Build history of the part. All positions in model axes, mm. Round coordinates to 2 decimals unless told otherwise and drop trailing zeros. Loops run counter-clockwise (first coordinate to the right, second up) from the corner with the lowest first, then second, coordinate; pieces in that order, holes last. Notation, with made-up numbers: (31.5, -39.5) - (78.5, -39.5) arc R20 cw to (78.5, -16.5) - close; hole circle Ø1 at (6.5, 76). An arc over 180 degrees is marked (long way). Use one line per item in the form item = value. Start each with the question number.
Q1. Drill centre lines: line 1 (X direction, y = -116, z = 0.6); line 2 (Y direction, x = 55, z = 0.75); line 3 (Y direction, x = 65, z = 1.3). Where is each one in solid material? Low to high.
Q2. Saw through at A-A (x = 65). Give the cut face in (y, z), then the cut area to 3 significant figures.
Q3. Pin check, flat tips, straight feed: pin 1 (9 mm diameter, centred on x = 65, y = -70, fed in from +Z); pin 2 (4.5 mm diameter, centred on x = 55, y = -116, fed in from +Z). Stop position of each tip, or through.
Autodesk Inventor part; units mm, degrees
ref_plane "YZ Plane" through (0, 0, 0) normal (1, 0, 0) x (0, 1, 0)
ref_plane "XZ Plane" through (0, 0, 0) normal (0, 1, 0) x (-1, 0, 0)
ref_plane "XY Plane" through (0, 0, 0) normal (0, 0, 1) x (1, 0, 0)
sketch "スケッチ1" plane through (0, 0, 0) normal (0, 0, 1) x (1, 0, 0)
  line L0 (0, 0) -> (360, 0)
  line L1 (360, 0) -> (360, -180)
  line L2 (360, -180) -> (0, -180)
  line L3 (0, -180) -> (0, 0)
  dimension "d0" = 360
  dimension "d1" = 180
extrude "押し出し1" add sketch "スケッチ1" along normal blind 2
sketch "スケッチ3" plane through (0, 0, 2) normal (0, 0, 1) x (1, 0, 0)
  line L0 (360, 0) -> (0, 0)
  line L1 (0, 0) -> (0, -180)
  point P0 (55, -139)
  point P1 (30, -139)
  point P2 (55, -116)
  point P3 (30, -116)
  dimension "d14" = 139
  dimension "d15" = 55
  dimension "d18" = 25
  dimension "d21" = 23
hole "穴2" at (55, -139, 2) at (30, -139, 2) at (55, -116, 2) at (30, -116, 2) direction (0, 0, -1) diameter 3.5 end through all
sketch "スケッチ4" plane through (0, 0, 0) normal (0, 0, -1) x (-1, 0, 0)
  line L0 (-360, 0) -> (0, 0)
  line L1 (0, 0) -> (0, -180)
  point P0 (-65, -70)
  dimension "d31" = 70
  dimension "d32" = 65
hole "穴3" at (65, -70, 0) direction (0, 0, 1) diameter 11 end through all
properties part number "後ろカバー" material "ABS プラスチック"
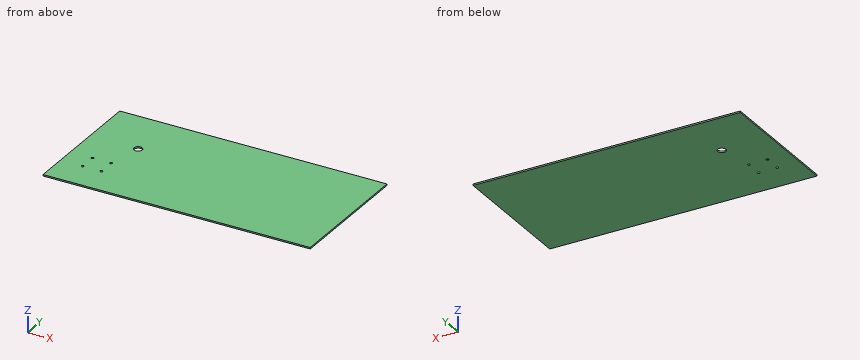
Report:
q1.line_1 = 0 to 28.25, 31.75 to 53.25, 56.75 to 360
q1.line_2 = -180 to -140.75, -137.25 to -117.75, -114.25 to 0
q1.line_3 = -180 to -75.5, -64.5 to 0
q2.outline = (-180, 0) - (-75.5, 0) - (-75.5, 2) - (-180, 2) - close; (-64.5, 0) - (0, 0) - (0, 2) - (-64.5, 2) - close
q2.area = 338 mm²
q3.pin_1 = through
q3.pin_2 = 2
